```python
from build123d import *

# Parameters (mm, degrees)
SKETCH_W     = 100
SKETCH_H     = 23.5
SKETCH_R     = 1.75
SKETCH_W_2   = 2
SKETCH_H_2   = 7
SKETCH_W_3   = 3.333334
SKETCH_H_3   = 4
SKETCH_W_4   = 3.333333
PAD_DEPTH    = 2
SKETCH001_W  = 51
SKETCH001_H  = 20.3
PAD001_DEPTH = 5


with BuildPart() as part:
    # Sketch → Pad (new body)
    with BuildSketch(Plane.XY):
        with Locations((0, 0.75)):
            Rectangle(SKETCH_W, SKETCH_H)
        with Locations((-45, 0)):
            Circle(SKETCH_R, mode=Mode.SUBTRACT)
        with Locations((45, 0)):
            Circle(SKETCH_R, mode=Mode.SUBTRACT)
        Polygon((-39.999987, 8.970025), (-29.999987, 8.970025), (-29.999987, 4.970025), (-33.33332, 4.970025), (-33.33332, 1.636691), (-36.666654, 1.636691), (-36.666654, 4.970025), (-39.999987, 4.970025), align=None, mode=Mode.SUBTRACT)
        with Locations((-39.999987, -0.029975)):
            Rectangle(SKETCH_W_2, SKETCH_H_2, mode=Mode.SUBTRACT)
        with Locations((-29.999987, -0.029975)):
            Rectangle(SKETCH_W_2, SKETCH_H_2, mode=Mode.SUBTRACT)
        Polygon((-22.499994, 8.985012), (-12.499994, 8.985012), (-12.499994, 4.985012), (-15.833327, 4.985012), (-15.833327, 1.651679), (-19.16666, 1.651679), (-19.16666, 4.985012), (-22.499994, 4.985012), align=None, mode=Mode.SUBTRACT)
        with Locations((-22.499994, -0.014988)):
            Rectangle(SKETCH_W_2, SKETCH_H_2, mode=Mode.SUBTRACT)
        with Locations((-12.499994, -0.014988)):
            Rectangle(SKETCH_W_2, SKETCH_H_2, mode=Mode.SUBTRACT)
        Polygon((-5, 9), (5, 9), (5, 5), (1.666667, 5), (1.666667, 1.666667), (-1.666667, 1.666667), (-1.666667, 5), (-5, 5), align=None, mode=Mode.SUBTRACT)
        with Locations((-5, 0)):
            Rectangle(SKETCH_W_2, SKETCH_H_2, mode=Mode.SUBTRACT)
        with Locations((5, 0)):
            Rectangle(SKETCH_W_2, SKETCH_H_2, mode=Mode.SUBTRACT)
        Polygon((12.499994, 9.014988), (22.499994, 9.014988), (22.499994, 5.014988), (19.16666, 5.014988), (19.16666, 1.681654), (15.833327, 1.681654), (15.833327, 5.014988), (12.499994, 5.014988), align=None, mode=Mode.SUBTRACT)
        with Locations((12.499994, 0.014988)):
            Rectangle(SKETCH_W_2, SKETCH_H_2, mode=Mode.SUBTRACT)
        with Locations((22.499994, 0.014988)):
            Rectangle(SKETCH_W_2, SKETCH_H_2, mode=Mode.SUBTRACT)
        Polygon((29.999987, 9.029975), (39.999987, 9.029975), (39.999987, 5.029975), (36.666654, 5.029975), (36.666654, 1.696642), (33.33332, 1.696642), (33.33332, 5.029975), (29.999987, 5.029975), align=None, mode=Mode.SUBTRACT)
        with Locations((29.999987, 0.029975)):
            Rectangle(SKETCH_W_2, SKETCH_H_2, mode=Mode.SUBTRACT)
        with Locations((39.999987, 0.029975)):
            Rectangle(SKETCH_W_2, SKETCH_H_2, mode=Mode.SUBTRACT)
        with Locations((34.999987, -3.636691)):
            Rectangle(SKETCH_W_3, SKETCH_H_3, mode=Mode.SUBTRACT)
        with Locations((-34.999987, -3.696642)):
            Rectangle(SKETCH_W_3, SKETCH_H_3, mode=Mode.SUBTRACT)
        with Locations((-17.499993, -3.681654)):
            Rectangle(SKETCH_W_4, SKETCH_H_3, mode=Mode.SUBTRACT)
        with Locations((0, -3.666667)):
            Rectangle(SKETCH_W_3, SKETCH_H_3, mode=Mode.SUBTRACT)
        with Locations((17.499993, -3.651679)):
            Rectangle(SKETCH_W_4, SKETCH_H_3, mode=Mode.SUBTRACT)
    extrude(amount=PAD_DEPTH)

    # Sketch001 → Pad001 (join)
    with BuildSketch(Plane.XY):
        Polygon((-50, 12.5), (-50, 10.9), (-27.1, 10.9), (-27.1, -9.4), (-50, -9.4), (-50, -11), (50, -11), (50, -9.4), (27.1, -9.4), (27.1, 10.9), (50, 10.9), (50, 12.5), align=None)
        with Locations((0, 0.75)):
            Rectangle(SKETCH001_W, SKETCH001_H, mode=Mode.SUBTRACT)
    extrude(amount=PAD001_DEPTH)


solid = part.part
```
The listing builds one solid part. Answer for the finished solid, in the listing's coordinates (mm). A direction names the side the tool comes from. Give positions to 0.01 mm unless a question says otherwise; leave off trailing zeros. Order: outer loops, then holes, each group sorted by start corner. A loop starts at its lowest first (then second) coordinate and runs counter-clockwise, first axis right, second up. Notation, with made-up numbers: (37.25, 28.25) - (89.25, 28.25) arc R13 ccw to (89.25, 41.25) - close; hole circle Ø1 at (-21, 1.5). An arc over 180 degrees is marked (long way). Answer in a Markdown table with one row per item. Add a question column.
Q1. Given P1, Ø4, axis at x = -45, y = 0, coming from the -Z side, flat-ended and moving along its own axis, determine where the tip first touches the part or whether it passes through.
Q2. Find the intervals of material crossed by line 1 along Y through (x, z) = (-17.5, 0.9); line 2 along X through (y, z) = (8, 1.75); line 3 along Y through (x, z) = (45, 1.55), in increasing order. Write a range as [from, to].
Q3. Which of the six approach directions +Z, -Z, +X, -X, +Y, -Y give full straight-line access (tool end or side, diameter ignored) to faces 5 (the flat face through (-19.167, 3, 1)), 6 (the flat face through (25.5, 1, 3))?
Q4. The part is cut by section A-A (x = 45). Determine the outline of the cut face in (y, z).
Q5. The part is cut by section B-B (y = 0). Give the number of separate pieces and of enclosed holes in the cut face, then the cut area to 3 significant figures.
Q6. The part is cut by section C-C (y = -7.25). Determine the outline of the cut face in (x, z), then the cut area to 3 significant figures.
Q7. For a pull along X with two mould halves and no side action, classify faces 1 (the flat face through (-22.5, 7, 1)), 2 (the flat face through (-38, -9.4, 3)), 3 (the flat face through (30, 3.53, 1)), 4 (the flat face through (50, 1, 1)) as released by +X, released by -X, zero draft, split by the parting line, or undercut.
Determined:
| question | item | result |
|---|---|---|
| 1 | P1 | stops at z = 0 |
| 2 | line 1 | y = [-11, -5.68], [-1.68, 1.65], [8.99, 12.5] |
| 2 | line 2 | x = [-50, -40], [-30, -22.5], [-12.5, -5], [5, 12.5], [22.5, 30], [40, 50] |
| 2 | line 3 | y = [-11, -1.75], [1.75, 12.5] |
| 3 | face 5 | +Z, -Z |
| 3 | face 6 | +Z |
| 4 | outline | (-11, 0) - (-1.75, 0) - (-1.75, 2) - (-9.4, 2) - (-9.4, 5) - (-11, 5) - close; (1.75, 0) - (12.5, 0) - (12.5, 5) - (10.9, 5) - (10.9, 2) - (1.75, 2) - close |
| 5 | separate pieces | 13 |
| 5 | enclosed holes | 0 |
| 5 | area | 156 mm² |
| 6 | outline | (-50, 0) - (50, 0) - (50, 2) - (27.1, 2) - (27.1, 5) - (25.5, 5) - (25.5, 2) - (-25.5, 2) - (-25.5, 5) - (-27.1, 5) - (-27.1, 2) - (-50, 2) - close |
| 6 | area | 210 mm² |
| 7 | face 1 | undercut |
| 7 | face 2 | zero draft |
| 7 | face 3 | undercut |
| 7 | face 4 | released by +X |
